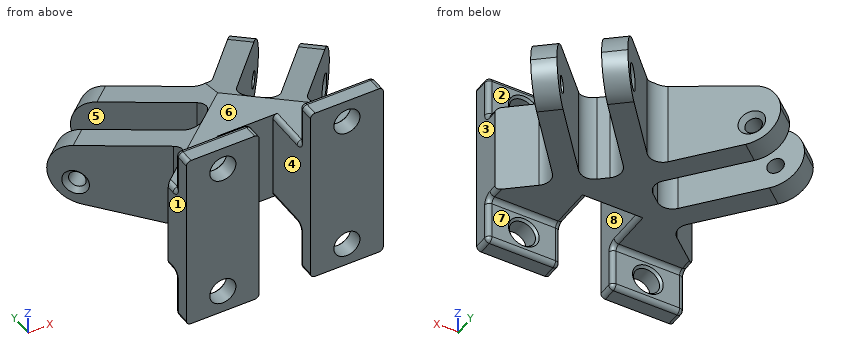
from build123d import *

# Parameters (mm, degrees)
BOSS_EXTRUDE1_DEPTH = 20
SKETCH5_R           = 1.75
CUT_EXTRUDE3_DEPTH  = 55.933306211
SKETCH6_R           = 1.75
CUT_EXTRUDE4_DEPTH  = 55.933306211
CUT_EXTRUDE5_DEPTH  = 55.933306211
CUT_EXTRUDE6_DEPTH  = 55.933306211
BOSS_EXTRUDE3_DEPTH = 10
SKETCH10_R          = 2.85
CUT_EXTRUDE7_DEPTH  = 4.933726003
BOSS_EXTRUDE4_DEPTH = 10
SKETCH12_R          = 2.85
CUT_EXTRUDE8_DEPTH  = 4.933726003
CUT_EXTRUDE9_DEPTH  = 41
CHAMFER1_SIZE       = 1
CHAMFER2_SIZE       = 0.5
FILLET1_R           = 1
FILLET2_R           = 3


with BuildPart() as part:
    # Sketch1 → Boss-Extrude1 (new body)
    with BuildSketch(Plane.XY):
        Polygon((-16.499999997, 0), (-0.605600394, 0), (-0.605600394, 13.845143912), (10.605600394, 13.845143912), (10.605600394, 0), (26.499999997, 0), (29.800788035, 3.933726003), (17.736610648, 14.0567728), (35.86606285, 35.662612593), (32.035840635, 38.876550642), (13.906388432, 17.270710848), (7.395010666, 22.73440553), (25.524462868, 44.340245324), (21.694240652, 47.554183373), (5, 27.658762099), (-11.694240652, 47.554183373), (-15.524462868, 44.340245324), (2.604989334, 22.73440553), (-3.906388432, 17.270710848), (-22.035840635, 38.876550642), (-25.86606285, 35.662612593), (-7.736610648, 14.0567728), (-19.800788035, 3.933726003), align=None)
    extrude(amount=BOSS_EXTRUDE1_DEPTH)

    # Sketch5 → Cut-Extrude3 (cut, through all)
    with BuildSketch(Plane(origin=(2.381579924, 1.998382835, 0), x_dir=(0, 0, 1), z_dir=(-0.766044443, -0.64278761, 0))):
        with Locations((5.02612125, 38.193531526)):
            Circle(SKETCH5_R)
    extrude(amount=-CUT_EXTRUDE3_DEPTH, mode=Mode.SUBTRACT)

    # Sketch6 → Cut-Extrude4 (cut, through all)
    with BuildSketch(Plane(origin=(3.486660965, -2.92565593, 0), x_dir=(0, 0, -1), z_dir=(0.766044443, -0.64278761, 0))):
        with Locations((-5.02612125, 44.621407623)):
            Circle(SKETCH6_R)
    extrude(amount=-CUT_EXTRUDE4_DEPTH, mode=Mode.SUBTRACT)

    # Sketch7 → Cut-Extrude5 (cut, through all)
    with BuildSketch(Plane(origin=(2.381579924, 1.998382835, 0), x_dir=(0, 0, 1), z_dir=(-0.766044443, -0.64278761, 0))):
        with BuildLine():
            ThreePointArc((0, 36.945530916), (2.050252532, 41.895278384), (7, 43.945530916))
            Line((7, 43.945530916), (0, 43.945530916))
            Line((0, 43.945530916), (0, 36.945530916))
        make_face()
        with BuildLine():
            ThreePointArc((7, 43.945530916), (11.317943157, 42.479786722), (13.851309254, 38.688336422))
            Line((13.851309254, 38.688336422), (20, 15.741110157))
            Line((20, 15.741110157), (20, 43.945530916))
            Line((20, 43.945530916), (7, 43.945530916))
        make_face()
    extrude(amount=-CUT_EXTRUDE5_DEPTH, mode=Mode.SUBTRACT)

    # Sketch8 → Cut-Extrude6 (cut, through all)
    with BuildSketch(Plane(origin=(3.486660965, -2.92565593, 0), x_dir=(0, 0, -1), z_dir=(0.766044443, -0.64278761, 0))):
        with BuildLine():
            Line((-20, 22.168986254), (-13.851309254, 45.116212519))
            ThreePointArc((-13.851309254, 45.116212519), (-11.317943157, 48.907662818), (-7, 50.373407013))
            Line((-7, 50.373407013), (-20, 50.373407013))
            Line((-20, 50.373407013), (-20, 22.168986254))
        make_face()
        with BuildLine():
            Line((0, 50.373407013), (-7, 50.373407013))
            ThreePointArc((-7, 50.373407013), (-2.050252532, 48.323154481), (0, 43.373407013))
            Line((0, 43.373407013), (0, 50.373407013))
        make_face()
    extrude(amount=-CUT_EXTRUDE6_DEPTH, mode=Mode.SUBTRACT)

    # Sketch9 → Boss-Extrude3 (add)
    with BuildSketch(Plane.XY.offset(20)):
        Polygon((-0.605600394, 0), (-16.499999997, 0), (-19.800788035, 3.933726003), (-0.605600394, 3.933726003), align=None)
        Polygon((10.605600394, 3.933726003), (10.605600394, 0), (26.499999997, 0), (29.800788035, 3.933726003), align=None)
    extrude(amount=BOSS_EXTRUDE3_DEPTH)

    # Sketch10 → Cut-Extrude7 (cut, through all)
    with BuildSketch(Plane(origin=(0, 3.933726003, 0), x_dir=(1, 0, 0), z_dir=(0, 1, 0))):
        with Locations((-8.552800195, -25)):
            Circle(SKETCH10_R)
        with Locations((18.552800195, -25)):
            Circle(SKETCH10_R)
    extrude(amount=-CUT_EXTRUDE7_DEPTH, mode=Mode.SUBTRACT)

    # Sketch11 → Boss-Extrude4 (add)
    with BuildSketch(Plane(origin=(0, 0, 0), x_dir=(-1, 0, 0), z_dir=(0, 0, -1))):
        Polygon((19.800788035, 3.933726003), (16.499999997, 0), (0.605600394, 0), (0.605600394, 3.933726003), align=None)
        Polygon((-10.605600394, 3.933726003), (-10.605600394, 0), (-26.499999997, 0), (-29.800788035, 3.933726003), align=None)
    extrude(amount=BOSS_EXTRUDE4_DEPTH)

    # Sketch12 → Cut-Extrude8 (cut, through all)
    with BuildSketch(Plane(origin=(0, 3.933726003, 0), x_dir=(1, 0, 0), z_dir=(0, 1, 0))):
        with Locations((-8.552800195, 5)):
            Circle(SKETCH12_R)
        with Locations((18.552800195, 5)):
            Circle(SKETCH12_R)
    extrude(amount=-CUT_EXTRUDE8_DEPTH, mode=Mode.SUBTRACT)

    # Sketch13 → Cut-Extrude9 (cut, through all)
    with BuildSketch(Plane.XY.offset(30)):
        Polygon((-16.499999997, 0), (-16.499999997, 3.933726003), (-16.499999997, 6.703416029), (-19.800788035, 3.933726003), align=None)
        Polygon((26.499999997, 0), (26.499999997, 3.933726003), (26.499999997, 6.703416029), (29.800788035, 3.933726003), align=None)
    extrude(amount=-CUT_EXTRUDE9_DEPTH, mode=Mode.SUBTRACT)

    # Chamfer1
    chamfer1_edges = [part.edges().sort_by_distance(p)[0] for p in [
        (17.996926714, 43.147896203, 6.77612125),
        (32.168748911, 31.256325424, 6.77612125),
        (-7.996926714, 43.147896203, 3.27612125),
        (-22.168748911, 31.256325424, 3.27612125),
    ]]
    chamfer(chamfer1_edges, length=CHAMFER1_SIZE)

    # Chamfer2
    chamfer2_edges = [part.edges().sort_by_distance(p)[0] for p in [
        (-11.402800195, 3.933726003, 25),
        (15.702800195, 3.933726003, 25),
        (15.702800195, 3.933726003, -5),
        (-11.402800195, 3.933726003, -5),
    ]]
    chamfer(chamfer2_edges, length=CHAMFER2_SIZE)

    # Fillet1
    fillet1_edges = [part.edges().sort_by_distance(p)[0] for p in [
        (-0.605600394, 8.889434958, 20),
        (10.605600394, 8.889434958, 20),
        (-8.552800195, 3.933726003, 20),
        (-0.605600394, 3.933726003, 25),
        (-0.605600394, 1.966863002, 30),
        (-8.552800195, 3.933726003, 30),
        (10.605600394, 3.933726003, 25),
        (10.605600394, 1.966863002, 30),
        (-0.605600394, 3.933726003, -5),
        (-0.605600394, 1.966863002, -10),
        (18.552800195, 3.933726003, 0),
        (10.605600394, 3.933726003, -5),
        (18.552800195, 3.933726003, -10),
        (10.605600394, 1.966863002, -10),
        (10.605600394, 8.889434958, 0),
        (26.499999997, 1.966863002, -10),
        (-8.552800195, 3.933726003, -10),
        (-8.552800195, 3.933726003, 0),
        (18.552800195, 3.933726003, 30),
        (18.552800195, 3.933726003, 20),
        (26.499999997, 1.966863002, 30),
        (26.499999997, 5.318571016, 20),
        (26.499999997, 5.318571016, 0),
        (26.499999997, 3.933726003, -5),
        (26.499999997, 3.933726003, 25),
        (-0.605600394, 8.889434958, 0),
        (-16.499999997, 1.966863002, 30),
        (-16.499999997, 5.318571016, 20),
        (-16.499999997, 3.933726003, 25),
        (-16.499999997, 1.966863002, -10),
        (-16.499999997, 3.933726003, -5),
        (-16.499999997, 5.318571016, 0),
    ]]
    fillet(fillet1_edges, radius=FILLET1_R)

    # Fillet2
    fillet2_edges = [part.edges().sort_by_distance(p)[0] for p in [
        (5, 27.658762099, 9.700862486),
        (-7.736610648, 14.0567728, 10),
        (-3.906388432, 17.270710848, 10),
        (2.604989334, 22.73440553, 10),
        (7.395010666, 22.73440553, 10),
        (13.906388432, 17.270710848, 10),
        (17.736610648, 14.0567728, 10),
    ]]
    fillet(fillet2_edges, radius=FILLET2_R)


solid = part.part
Source: CAD feature listing. Evaluate the final solid. Frame: model axes, mm. Face numbers are marked on the shaded views. A direction names the side the tool comes from. Round coordinates to 2 decimals unless told otherwise and drop trailing zeros. Loops run counter-clockwise (first coordinate to the right, second up) from the corner with the lowest first, then second, coordinate; pieces in that order, holes last. Notation, with made-up numbers: M 6.25,14.5 L 16.25,14.5 A23 ccw 16.25,44.5 Z; hole C 48.5,-13.75 d10. An arc over 180 degrees is marked long. Return JSON: item names as keys, results as strings. Group by question number.
1. Section query A-A on z = 25. Output: boundary loops of the cut face in (x, y), and give its area (3 significant figures).
2. Section query D-D on z = -3. State how many separate pieces and enclosed holes the cut face has, and give its area (3 significant figures).
3. Mould query, pull axis X, two halves, no side actions, for the marked faces 1, 2, 3 and 4. Classes: released by +X, released by -X, zero draft, split by the parting line, or undercut.
4. Material intervals for line 1 along X through (y, z) = (2, -5); line 2 along X through (y, z) = (27, 11.5); line 3 along X through (y, z) = (37, 11), sorted ascending. Write a range as from..to.
5. Reachability of the marked faces 5, 6, 7 and 8 from +Z, -Z, +X, -X, +Y, -Y: full face, straight path, thin tool, end or side. Return the list, or none.
6. Pin query (flat end, axial travel): pin 1 (6 mm diameter, centred on y = 42, z = -1.5, fed in from +X); pin 2 (3 mm diameter, centred on x = 6.5, z = 22, fed in from +Y); pin 3 (1.5 mm diameter, centred on x = 0.5, y = 30.5, fed in from +Z); pin 4 (3 mm diameter, centred on x = 11, y = 15.5, fed in from +Z). Return the tip coordinate at first contact, or that it passes through.
7. Section query B-B on y = 11. Output: boundary loops of the cut face in (x, z), and give its area (3 significant figures).
Checks:
{
 "1": {"outline": "M -16.5,0 L -11.4,0 L -11.4,3.43 L -11.9,3.93 L -15.5,3.93 A1 ccw -16.5,2.93 Z; M -5.7,0 L -0.61,0 L -0.61,2.93 A1 ccw -1.61,3.93 L -5.2,3.93 L -5.7,3.43 Z; M 10.61,0 L 15.7,0 L 15.7,3.43 L 15.2,3.93 L 11.61,3.93 A1 ccw 10.61,2.93 Z; M 21.4,0 L 26.5,0 L 26.5,2.93 A1 ccw 25.5,3.93 L 21.9,3.93 L 21.4,3.43 Z", "area": "78.8 mm²"},
 "2": {"separate pieces": "4", "enclosed holes": "0", "area": "91.6 mm²"},
 "3": {"face 1": "released by -X", "face 2": "zero draft", "face 3": "released by +X", "face 4": "undercut"},
 "4": {"line 1": "x = -16.5..-11.4, -5.7..-0.61, 10.61..15.7, 21.4..26.5", "line 2": "x = -18.6..-12.07, -0.97..10.97, 22.07..28.6", "line 3": "x = -22.35..-20.46, -9.37..-2.84, 12.84..19.37, 30.46..32.35"},
 "5": {"face 5": "+Z, -Z", "face 6": "+Z, +X, -X, +Y", "face 7": "-Z, +X, -X, +Y", "face 8": "+Z, -Z, -Y"},
 "6": {"pin 1": "stops at x = 23.8", "pin 2": "passes through", "pin 3": "stops at z = 18.24", "pin 4": "stops at z = 20"},
 "7": {"outline": "M -11.38,0 L -1.61,0 A1 ccw -0.61,1 L -0.61,19 A1 ccw -1.61,20 L -11.38,20 Z; M 10.61,1 A1 ccw 11.61,0 L 21.38,0 L 21.38,20 L 11.61,20 A1 ccw 10.61,19 Z", "area": "430 mm²"}
}
